Work out the finished part from the listing and answer in its coordinate system (mm). Face numbers are marked on the shaded views. A direction names the side the tool comes from. Round coordinates to 2 decimals unless told otherwise and drop trailing zeros. Order: outer loops, then holes, each group sorted by start corner. A loop starts at its lowest first (then second) coordinate and runs counter-clockwise, first axis right, second up. Notation, with made-up numbers: (37, -24) - (65, -24) arc R23 cw to (65, -7) - close; hole circle Ø7 at (75, 7.25). An arc over 180 degrees is marked (long way). Put each result on its own line as item: value.
```python
from build123d import *

# Parameters (mm, degrees)
SKETCH_1_W          = 129
SKETCH_1_H          = 88.5
EXTRUDE_1_DEPTH     = 3
SKETCH_2_R          = 5.00000016
CUT_EXTRUDE_1_DEPTH = 154.829654163
SKETCH_3_R          = 1.6
CUT_EXTRUDE_2_DEPTH = 154.829654163
CHAMFER_1_SIZE      = 1
CHAMFER_2_SIZE      = 1
SKETCH_6_W          = 124.5
SKETCH_6_H          = 84.5
EXTRUDE_3_DEPTH     = 3.5
SKETCH_7_R          = 5.00000016
SKETCH_7_R_2        = 1.6
CUT_EXTRUDE_3_DEPTH = 154.840217434
SKETCH_9_R          = 12.5
CUT_EXTRUDE_4_DEPTH = 3.5
FILLET_4_R          = 1
FILLET_5_R          = 1
FILLET_6_R          = 1


with BuildPart() as part:
    # Эскиз1 → Бобышка-Вытянуть1 (new body)
    with BuildSketch(Plane(origin=(0, 37.5, 0), x_dir=(1, 0, 0), z_dir=(0, 1, 0))):
        with Locations((62.5, 42.5)):
            Rectangle(SKETCH_1_W, SKETCH_1_H)
    extrude(amount=EXTRUDE_1_DEPTH)

    # Эскиз2 → Вырез-Вытянуть1 (cut, through all)
    with BuildSketch(Plane(origin=(0, 40.5, 0), x_dir=(1, 0, 0), z_dir=(0, 1, 0))):
        with Locations(Location((43.5999659, 14.50003568, 0), (0, 0, 270))):
            Circle(SKETCH_2_R)
        with Locations(Location((43.5999659, 42.50003556, 0), (0, 0, 270))):
            Circle(SKETCH_2_R)
        with Locations(Location((68.5999667, 70.50003544, 0), (0, 0, 270))):
            Circle(SKETCH_2_R)
        with Locations(Location((93.5999675, 42.50003556, 0), (0, 0, 270))):
            Circle(SKETCH_2_R)
        with Locations(Location((93.5999675, 14.50003568, 0), (0, 0, 270))):
            Circle(SKETCH_2_R)
    extrude(amount=-CUT_EXTRUDE_1_DEPTH, mode=Mode.SUBTRACT)

    # Эскиз3 → Вырез-Вытянуть2 (cut, through all)
    with BuildSketch(Plane(origin=(0, 40.5, 0), x_dir=(1, 0, 0), z_dir=(0, 1, 0))):
        with Locations(Location((34.59981372, 80.23011504, 0), (0, 0, 270))):
            Circle(SKETCH_3_R)
        with Locations(Location((26.6000126, 80.22990168, 0), (0, 0, 270))):
            Circle(SKETCH_3_R)
        with Locations(Location((18.5998381, 80.23011504, 0), (0, 0, 270))):
            Circle(SKETCH_3_R)
        with Locations(Location((8.59981492, 41.2301143, 0), (0, 0, 270))):
            Circle(SKETCH_3_R)
        with Locations(Location((16.59981416, 41.2300889, 0), (0, 0, 270))):
            Circle(SKETCH_3_R)
        with Locations(Location((24.60001152, 41.22987554, 0), (0, 0, 270))):
            Circle(SKETCH_3_R)
        with Locations(Location((17.59991376, 5.79999466, 0), (0, 0, 270))):
            Circle(SKETCH_3_R)
        with Locations(Location((22.59991392, 5.79999466, 0), (0, 0, 270))):
            Circle(SKETCH_3_R)
        with Locations(Location((27.59991408, 5.79999466, 0), (0, 0, 270))):
            Circle(SKETCH_3_R)
    extrude(amount=-CUT_EXTRUDE_2_DEPTH, mode=Mode.SUBTRACT)

    # Фаска1
    chamfer_1_edges = [part.edges().sort_by_distance(p)[0] for p in [
        (43.5999659, 37.5, -19.50003584),
        (43.5999659, 37.5, -47.50003572),
        (68.5999667, 37.5, -75.5000356),
        (93.5999675, 37.5, -47.50003572),
        (93.5999675, 37.5, -19.50003584),
    ]]
    chamfer(chamfer_1_edges, length=CHAMFER_1_SIZE)

    # Фаска2
    chamfer_2_edges = [part.edges().sort_by_distance(p)[0] for p in [
        (34.59981372, 37.5, -81.83011504),
        (26.6000126, 37.5, -81.82990168),
        (18.5998381, 37.5, -81.83011504),
        (8.59981492, 37.5, -42.8301143),
        (16.59981416, 37.5, -42.8300889),
        (24.60001152, 37.5, -42.82987554),
    ]]
    chamfer(chamfer_2_edges, length=CHAMFER_2_SIZE)

    # Эскиз6 → Бобышка-Вытянуть3 (add)
    with BuildSketch(Plane(origin=(0, 40.5, 0), x_dir=(1, 0, 0), z_dir=(0, 1, 0))):
        with Locations((62.5, 42.5)):
            Rectangle(SKETCH_6_W, SKETCH_6_H)
    extrude(amount=EXTRUDE_3_DEPTH)

    # Эскиз7 → Вырез-Вытянуть3 (cut, through all)
    with BuildSketch(Plane.XZ.offset(-40.5)):
        with Locations(Location((43.5999659, -42.50003556, 0), (0, 0, 90))):
            Circle(SKETCH_7_R)
        with Locations(Location((43.5999659, -14.50003568, 0), (0, 0, 90))):
            Circle(SKETCH_7_R)
        with Locations(Location((93.5999675, -14.50003568, 0), (0, 0, 90))):
            Circle(SKETCH_7_R)
        with Locations(Location((93.5999675, -42.50003556, 0), (0, 0, 90))):
            Circle(SKETCH_7_R)
        with Locations(Location((68.5999667, -70.50003544, 0), (0, 0, 90))):
            Circle(SKETCH_7_R)
        with Locations(Location((24.60001152, -41.22987554, 0), (0, 0, 90))):
            Circle(SKETCH_7_R_2)
        with Locations(Location((16.59981416, -41.2300889, 0), (0, 0, 90))):
            Circle(SKETCH_7_R_2)
        with Locations(Location((8.59981492, -41.2301143, 0), (0, 0, 90))):
            Circle(SKETCH_7_R_2)
        with Locations(Location((18.5998381, -80.23011504, 0), (0, 0, 90))):
            Circle(SKETCH_7_R_2)
        with Locations(Location((26.6000126, -80.22990168, 0), (0, 0, 90))):
            Circle(SKETCH_7_R_2)
        with Locations(Location((34.59981372, -80.23011504, 0), (0, 0, 90))):
            Circle(SKETCH_7_R_2)
        with Locations(Location((17.59991376, -5.79999466, 0), (0, 0, 90))):
            Circle(SKETCH_7_R_2)
        with Locations(Location((22.59991392, -5.79999466, 0), (0, 0, 90))):
            Circle(SKETCH_7_R_2)
        with Locations(Location((27.59991408, -5.79999466, 0), (0, 0, 90))):
            Circle(SKETCH_7_R_2)
    extrude(amount=-CUT_EXTRUDE_3_DEPTH, mode=Mode.SUBTRACT)

    # Эскиз9 → Вырез-Вытянуть4 (cut)
    with BuildSketch(Plane(origin=(0, 44, 0), x_dir=(1, 0, 0), z_dir=(0, 1, 0))):
        with Locations(Location((43.5999659, 14.50003568, 0), (0, 0, 270))):
            Circle(SKETCH_9_R)
        with Locations(Location((43.5999659, 42.50003556, 0), (0, 0, 270))):
            Circle(SKETCH_9_R)
        with Locations(Location((68.5999667, 70.50003544, 0), (0, 0, 270))):
            Circle(SKETCH_9_R)
        with Locations(Location((93.5999675, 42.50003556, 0), (0, 0, 270))):
            Circle(SKETCH_9_R)
        with Locations(Location((93.5999675, 14.50003568, 0), (0, 0, 270))):
            Circle(SKETCH_9_R)
    extrude(amount=-CUT_EXTRUDE_4_DEPTH, mode=Mode.SUBTRACT)

    # Скругление4
    fillet_4_edges = [part.edges().sort_by_distance(p)[0] for p in [
        (124.75, 42.25, -0.25),
        (124.75, 42.25, -84.75),
        (127, 39, 1.75),
        (127, 39, -86.75),
    ]]
    fillet(fillet_4_edges, radius=FILLET_4_R)

    # Скругление5
    fillet_5_edges = [part.edges().sort_by_distance(p)[0] for p in [
        (62, 40.5, 1.75),
        (127, 40.5, -42.5),
        (62, 40.5, -86.75),
        (126.707106781, 40.5, -86.457106781),
        (126.707106781, 40.5, 1.457106781),
    ]]
    fillet(fillet_5_edges, radius=FILLET_5_R)

    # Скругление6
    fillet_6_edges = [part.edges().sort_by_distance(p)[0] for p in [
        (-2, 40.5, -42.5),
        (-2, 38.5, 1.75),
        (-2, 38.5, -86.75),
        (-2, 40.207106781, -86.457106781),
        (-2, 40.207106781, 1.457106781),
    ]]
    fillet(fillet_6_edges, radius=FILLET_6_R)


solid = part.part
```
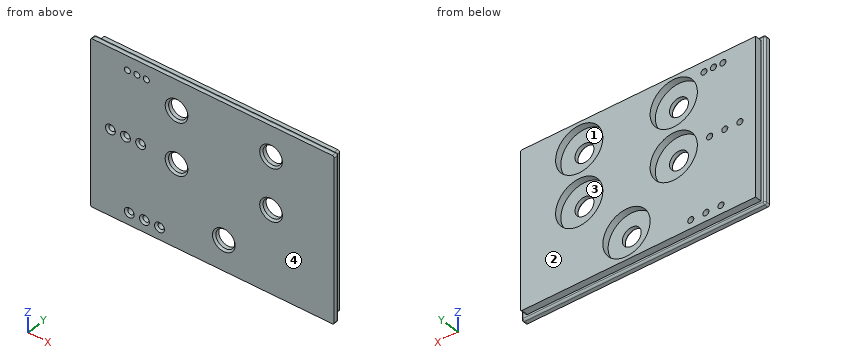
1) A cutting plane is placed at B-B on x = 84.5. Write down the section's boundary in (y, z).
Findings below:
outline: (37.5, -86.75) - (39.5, -86.75) arc R1 ccw to (40.5, -85.75) - (40.5, -84.75) - (44, -84.75) - (44, -51.07) - (40.5, -51.07) - (40.5, -33.93) - (44, -33.93) - (44, -23.07) - (40.5, -23.07) - (40.5, -5.93) - (44, -5.93) - (44, -0.25) - (40.5, -0.25) - (40.5, 0.75) arc R1 ccw to (39.5, 1.75) - (37.5, 1.75) - close
2) Given pin 1 Ø3 at (x, y) = (34.5, 42.5) entering from -Z; pin 2 Ø4 at (x, z) = (8.6, -41.23) entering from +Y; pin 3 Ø9 at (x, z) = (43.6, -14.5) entering from +Y; pin 4 Ø3.5 at (x, z) = (34.6, -80.23) entering from -Y, each flat-ended and moving along its own axis, determine where each tip first touches the part or whether it passes through.
Findings below:
pin 1: stops at z = -84.75
pin 2: stops at y = 44
pin 3: passes through
pin 4: stops at y = 38.35
3) For a pull along X with two mould halves and no side action, classify the marked faces 3 and 4 as pulls with the +X half, pulls with the -X half, needs draft (parallel to the pull), parting line crosses it, or undercut.
Findings below:
face 3: undercut
face 4: needs draft
4) A cutting plane is placed at D-D on z = -32.5. Write down the section's boundary in (x, y).
Findings below:
outline: (-2, 37.5) - (127, 37.5) - (127, 39.5) arc R1 ccw to (126, 40.5) - (124.75, 40.5) - (124.75, 44) - (101.1, 44) - (101.1, 40.5) - (86.1, 40.5) - (86.1, 44) - (51.1, 44) - (51.1, 40.5) - (36.1, 40.5) - (36.1, 44) - (0.25, 44) - (0.25, 40.5) - (-1, 40.5) arc R1 ccw to (-2, 39.5) - close
5) For the marked faces 1 and 2, determine the directions among +Z, -Z, +X, -X, +Y, -Y from which every point of the face is accessible in a straight line to the end or side of a thin tool.
Findings below:
face 1: +Y
face 2: +Z, -Z, +X, -X, +Y
6) A cutting plane is placed at A-A on z = -5.5. Give the number of separate pieces and of enclosed holes in the cut face, then the cut area to 3 significant figures.
Findings below:
separate pieces: 4
enclosed holes: 0
area: 640 mm2
7) Straight lines are drawn through the part: L1, parallel to X at y = 40.75, z = -14.5; L2, parallel to X at y = 39.5, z = -15; L3, parallel to X at y = 42.5, z = -41. For each, find the intervals that lie inside material, in ascending order. Write a range as from..to.
Findings below:
L1: x = 0.25..31.1, 56.1..81.1, 106.1..124.75
L2: x = -2..38.63, 48.57..88.63, 98.57..127
L3: x = 0.25..7.02, 10.18..15.02, 18.18..23.02, 26.18..31.19, 56.01..81.19, 106.01..124.75
